```python
from build123d import *

# Parameters (mm, degrees)
BOSS_EXTRUDE1_DEPTH = 203.5175
FILLET1_R           = 1.016


with BuildPart() as part:
    # Sketch2 → Boss-Extrude1 (new body)
    with BuildSketch(Plane.XY):
        with BuildLine():
            Line((-6.735192091, -6.735192091), (-13.470384182, 0))
            Line((-13.470384182, 0), (-14.188804671, -0.71842049))
            Line((-14.188804671, -0.71842049), (-6.735192091, -8.17203307))
            Line((-6.735192091, -8.17203307), (-1.412145275, -2.848986254))
            ThreePointArc((-1.412145275, -2.848986254), (-1.394184763, -2.848986254), (-1.394184763, -2.866946767))
            Line((-1.394184763, -2.866946767), (-6.717231579, -8.189993582))
            ThreePointArc((-6.717231579, -8.189993582), (0.574505978, -10.754978809), (7.655668343, -7.655668343))
            Line((7.655668343, -7.655668343), (0.359210245, -0.359210245))
            Line((0.359210245, -0.359210245), (7.094402336, 6.375981846))
            Line((7.094402336, 6.375981846), (6.375981846, 7.094402336))
            Line((6.375981846, 7.094402336), (-1.077630735, -0.359210245))
            Line((-1.077630735, -0.359210245), (6.182455958, -7.619296938))
            ThreePointArc((6.182455958, -7.619296938), (0.578453997, -9.738038748), (-5.182039359, -8.091642343))
            Line((-5.182039359, -8.091642343), (-0.675764273, -3.585367256))
            ThreePointArc((-0.675764273, -3.585367256), (-0.675764273, -2.130565765), (-2.130565765, -2.130565765))
            Line((-2.130565765, -2.130565765), (-6.735192091, -6.735192091))
        make_face()
    extrude(amount=-BOSS_EXTRUDE1_DEPTH)

    # Fillet1
    fillet1_edges = [part.edges().sort_by_distance(p)[0] for p in [
        (-1.077630735, -0.359210245, -101.75875),
        (7.655668343, -7.655668343, -101.75875),
        (-6.717231579, -8.189993582, -101.75875),
        (-6.735192091, -8.17203307, -101.75875),
    ]]
    fillet(fillet1_edges, radius=FILLET1_R)


solid = part.part
```
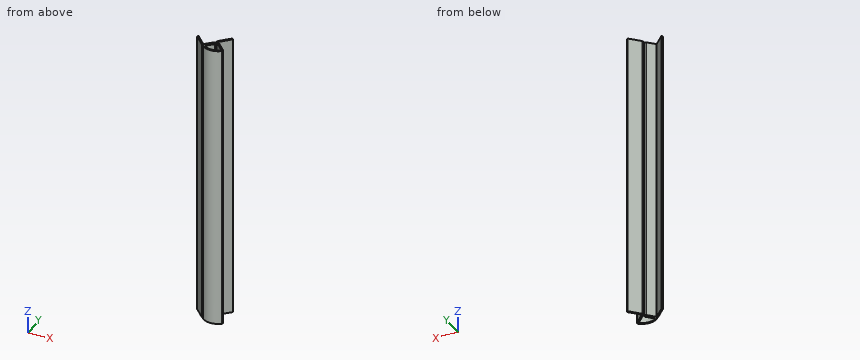
Model file for the job. Use its own axes, mm. Coordinates: 2 decimals unless noted, no trailing zeros. Order: outer loops, then holes, each group sorted by start corner. A loop starts at its lowest first (then second) coordinate and runs counter-clockwise, first axis right, second up. Notation, with made-up numbers: M 42.25,38 L 50.25,38 A23 ccw 50.25,65 Z; hole C -32,-26.75 d8. An arc over 180 degrees is marked long. Answer as CSV lines item,"result".
(1) Band-saw the part on A-A, the plane z = -92. List the corners of the cut face in (x, y) (3 decimals).
Geometry says:
outline,"M -14.189,-0.718 L -7.454,-7.454 A1.016 ccw -6.017,-7.454 L -1.412,-2.849 A0.013 cw -1.394,-2.867 L -5.9,-7.373 A1.016 ccw -5.754,-8.931 A10.541 ccw 6.822,-8.408 A1.016 ccw 6.901,-6.901 L 0.359,-0.359 L 7.094,6.376 L 6.376,7.094 L -0.359,0.359 A1.016 ccw -0.359,-1.078 L 6.182,-7.619 A9.525 cw -5.182,-8.092 L -0.676,-3.585 A1.029 ccw -2.131,-2.131 L -6.735,-6.735 L -13.47,0 Z"
(2) Wall check: line 1 along Y through (x, z) = (6, -42); line 2 along Y through (x, z) = (4.5, -173); line 3 along X through (y, z) = (-0.75, -129). Give the ranges that are in metal, low to high.
Geometry says:
line 1,"y = -9.01 to -7.76, -7.44 to -6, 5.28 to 6.72"
line 2,"y = -9.84 to -8.71, -5.94 to -4.5, 3.78 to 5.22"
line 3,"x = -14.16 to -12.72, -0.58 to 0.75"
(3) Band-saw the part on B-B, the plane x = 2.25. List the corners of the cut face in (y, z), then the cut area to 3 significant figures.
Geometry says:
outline,"M -10.56,-203.52 L -9.52,-203.52 L -9.52,0 L -10.56,0 Z; M -3.69,-203.52 L -2.25,-203.52 L -2.25,0 L -3.69,0 Z; M 1.53,-203.52 L 2.97,-203.52 L 2.97,0 L 1.53,0 Z"
area,"796 mm2"
(4) Flat gauge pins, fed straight in: pin 1 (4 mm diameter, centred on x = -6.5, z = -123.5, fed in from +Y); pin 2 (1 mm diameter, centred on x = 1.5, z = -156.5, fed in from +Y); pin 3 (6 mm diameter, centred on y = 0.5, z = -52, fed in from +X). Where does each tip first touch, or does it go through?
Geometry says:
pin 1,"stops at y = -4.5"
pin 2,"stops at y = 2.72"
pin 3,"stops at x = 4.22"
(5) Band-saw the part on C-C, the plane y = 3.25. List the corners of the cut face in (x, z).
Geometry says:
outline,"M 2.53,-203.52 L 3.97,-203.52 L 3.97,0 L 2.53,0 Z"
